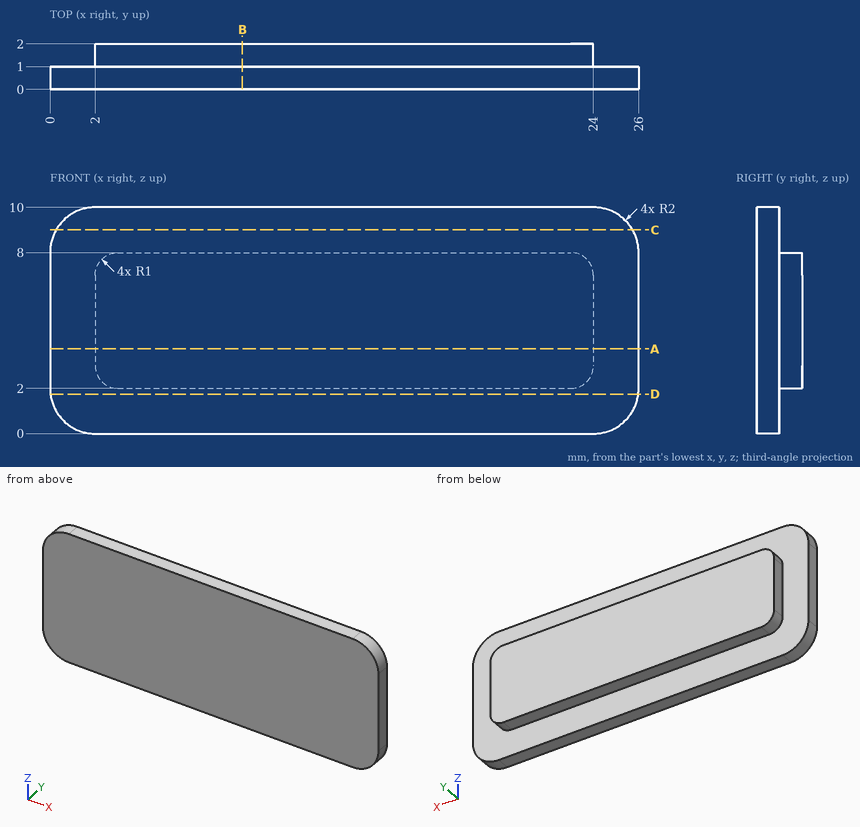
Design review of the part shown in the three views and the two pictorial views. Dimensions are in mm from the part's minimum x, y and z. Give positions to 0.01 mm unless a question says otherwise; leave off trailing zeros. Loops run counter-clockwise (first coordinate to the right, second up) from the corner with the lowest first, then second, coordinate; pieces in that order, holes last. Notation, with made-up numbers: (68, 55) -> (96, 55) arc R25 cw to (96, 75) -> close; hole circle Ø7 at (48.25, 64.25). An arc over 180 degrees is marked (long way). One line per question, with ' | ' between items.
1) We need section A-A (z = 3.75). Write out the cut boundary in (x, y), plus the area to 3 significant figures.
Resolved:
outline: (0, 0) -> (26, 0) -> (26, 1) -> (24, 1) -> (24, 2) -> (2, 2) -> (2, 1) -> (0, 1) -> close | area: 48.0 mm2
2) We need section D-D (z = 1.75). Write out the cut boundary in (x, y), plus the area to 3 significant figures.
Resolved:
outline: (0.02, 0) -> (25.98, 0) -> (25.98, 1) -> (0.02, 1) -> close | area: 26.0 mm2
3) To check wall thickness, follow probe 1 along Y at (x, z) = (20, 8.75); probe 2 along Z at (x, y) = (23, 1.7); probe 3 along X at (y, z) = (1.25, 3.75). State the ranges of each line that lie inside material, in increasing order.
Resolved:
probe 1: y = 0 to 1 | probe 2: z = 2 to 8 | probe 3: x = 2 to 24
4) We need section B-B (x = 8.5). Write out the cut boundary in (y, z).
Resolved:
outline: (0, 0) -> (1, 0) -> (1, 2) -> (2, 2) -> (2, 8) -> (1, 8) -> (1, 10) -> (0, 10) -> close
5) Insertion check: pin 1 Ø0.5 at (y, z) = (1.5, 4.5) entering from +X; pin 2 Ø0.5 at (x, y) = (8.5, 1.5) entering from +Z. Each pin has a flat end and moves straight along its axis. Give the tip position at first contact, or say it passes through.
Resolved:
pin 1: stops at x = 24 | pin 2: stops at z = 8
6) We need section C-C (z = 9). Write out the cut boundary in (x, y), plus the area to 3 significant figures.
Resolved:
outline: (0.27, 0) -> (25.73, 0) -> (25.73, 1) -> (0.27, 1) -> close | area: 25.5 mm2
